from build123d import *

# Parameters (mm, degrees)
BOSS_EXTRUDE1_DEPTH      = 3
SKETCH2_W                = 13
SKETCH2_H                = 23.5
BOSS_EXTRUDE2_DEPTH      = 4
SKETCH3_W                = 6
SKETCH3_H                = 1
BOSS_EXTRUDE3_DEPTH      = 6
CHAMFER1_SIZE            = 1
SKETCH4_W                = 19
SKETCH4_H                = 29.5
BOSS_EXTRUDE4_DEPTH      = 1.5
SKETCH5_W                = 10
SKETCH5_H                = 24
CUT_EXTRUDE1_DEPTH       = 1
BOSS_EXTRUDE5_DEPTH      = 4.9
BOSS_EXTRUDE5_DEPTH_BACK = 4.9
CHAMFER2_SIZE            = 1
CHAMFER2_SIZE2           = 0.754975442


with BuildPart() as part:
    # Sketch1 → Boss-Extrude1 (new body)
    with BuildSketch(Plane(origin=(0, 0, 0), x_dir=(1, 0, 0), z_dir=(0, 1, 0))):
        Polygon((0.75, -11.75), (6.5, -11.75), (6.5, 11.75), (0.75, 11.75), (0.75, 14), (-0.75, 14), (-0.75, 11.75), (-6.5, 11.75), (-6.5, -11.75), (-0.75, -11.75), (-0.75, -14), (0.75, -14), align=None)
    extrude(amount=-BOSS_EXTRUDE1_DEPTH)

    # Sketch2 → Boss-Extrude2 (add)
    with BuildSketch(Plane.XZ.offset(3)):
        Rectangle(SKETCH2_W, SKETCH2_H)
    extrude(amount=BOSS_EXTRUDE2_DEPTH)

    # Sketch3 → Boss-Extrude3 (add)
    with BuildSketch(Plane.XZ.offset(7)):
        Rectangle(SKETCH3_W, SKETCH3_H)
        with Locations((0, 6)):
            Rectangle(SKETCH3_W, SKETCH3_H)
        with Locations((0, -6)):
            Rectangle(SKETCH3_W, SKETCH3_H)
    extrude(amount=BOSS_EXTRUDE3_DEPTH)

    # Chamfer1
    chamfer1_edges = [part.edges().sort_by_distance(p)[0] for p in [
        (-3, -13, 0),
        (3, -13, 0),
        (-3, -13, 6),
        (3, -13, 6),
        (3, -13, -6),
        (-3, -13, -6),
    ]]
    chamfer(chamfer1_edges, length=CHAMFER1_SIZE)

    # Sketch4 → Boss-Extrude4 (add)
    with BuildSketch(Plane(origin=(0, 0, 0), x_dir=(1, 0, 0), z_dir=(0, 1, 0))):
        Rectangle(SKETCH4_W, SKETCH4_H)
    extrude(amount=BOSS_EXTRUDE4_DEPTH)

    # Sketch5 → Cut-Extrude1 (cut)
    with BuildSketch(Plane(origin=(0, 1.5, 0), x_dir=(1, 0, 0), z_dir=(0, 1, 0))):
        Rectangle(SKETCH5_W, SKETCH5_H)
    extrude(amount=-CUT_EXTRUDE1_DEPTH, mode=Mode.SUBTRACT)

    # Sketch6 → Boss-Extrude5 (add, two sides: drawn at the far end of the back side and taken through both)
    with BuildSketch(Plane(origin=(0, 0, 0), x_dir=(0, 0, -1), z_dir=(1, 0, 0)).offset(-BOSS_EXTRUDE5_DEPTH_BACK)):
        Polygon((-10.977846987, 0), (10.977846987, 0), (10.977846987, 2), (0, 2), (-10.977846987, 7), align=None)
    extrude(amount=BOSS_EXTRUDE5_DEPTH + BOSS_EXTRUDE5_DEPTH_BACK)

    # Chamfer2
    chamfer2_edges = [part.edges().sort_by_distance(p)[0] for p in [
        (0, 7, 10.977846987),
    ]]
    chamfer2_side = [part.faces().sort_by_distance(p)[0] for p in [
        (0, 3.75, 10.977846987),
    ]]
    chamfer(chamfer2_edges, length=CHAMFER2_SIZE, length2=CHAMFER2_SIZE2, reference=chamfer2_side[0])


solid = part.part
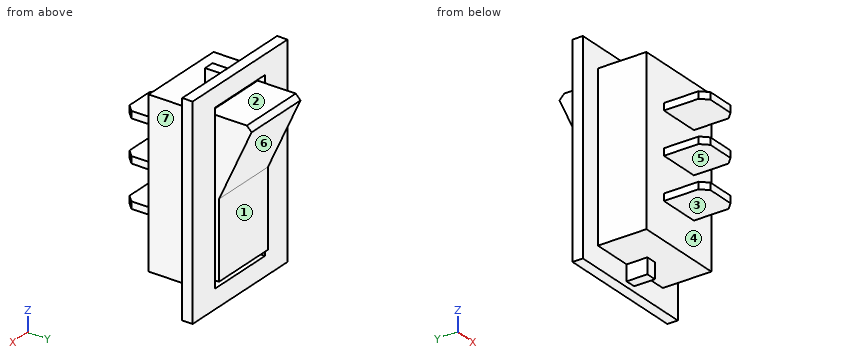
Model file for the job. Use its own axes, mm. Face numbers are marked on the shaded views. A direction names the side the tool comes from. Round coordinates to 2 decimals unless told otherwise and drop trailing zeros. Loops run counter-clockwise (first coordinate to the right, second up) from the corner with the lowest first, then second, coordinate; pieces in that order, holes last. Notation, with made-up numbers: (-20, 1.5) -> (17, 1.5) arc R20 ccw to (17, 40.5) -> close; hole circle Ø2 at (5, 79.5). An arc over 180 degrees is marked (long way). Answer as CSV lines item,"result". Start each with the question number.
1) Mould opens along Z. For the marked faces 4, 5, 6 and 7 say: +Z half, -Z half, draft (parallel to the pull), parting line (faces both ways), or undercut.
2) Slice it at D-D (y = -2.5). List the corners of the cut face in (x, z), plus the area to 3 significant figures.
3) Slice it at A-A (y = -7.75). List the corners of the cut face in (x, z), plus the area to 3 significant figures.
4) Pin check, flat tips, straight feed: P1, Ø6, axis at y = -7.5, z = -10, coming from the -X side; P2, Ø1.5, axis at y = -2.5, z = -9.5, coming from the +X side; P3, Ø5.5, axis at x = -2.5, y = -4.5, coming from the -Z side. Stop position of each tip, or through.
5) Probe line 1 along Y through (x, z) = (7.5, -2); line 2 along X through (y, z) = (-3, -6.75); line 3 along Z through (x, y) = (-0.75, -4.75). List the from-to ranges inside material, lowest first.
6) Slice it at C-C (z = -6). List the corners of the cut face in (x, y).
7) Tool access for the marked faces 1, 2 and 3: list every direction of +Z, -Z, +X, -X, +Y, -Y with a clear straight run to the whole face (end or side of a thin tool).
Filled in:
1,face 4,"undercut"
1,face 5,"undercut"
1,face 6,"-Z half"
1,face 7,"draft"
2,outline,"(-6.5, -11.75) -> (-0.75, -11.75) -> (-0.75, -14) -> (0.75, -14) -> (0.75, -11.75) -> (6.5, -11.75) -> (6.5, 11.75) -> (0.75, 11.75) -> (0.75, 14) -> (-0.75, 14) -> (-0.75, 11.75) -> (-6.5, 11.75) -> close"
2,area,"312 mm2"
3,outline,"(-3, -6.5) -> (3, -6.5) -> (3, -5.5) -> (-3, -5.5) -> close; (-3, -0.5) -> (3, -0.5) -> (3, 0.5) -> (-3, 0.5) -> close; (-3, 5.5) -> (3, 5.5) -> (3, 6.5) -> (-3, 6.5) -> close"
3,area,"18.0 mm2"
4,P1,"stops at x = -6.5"
4,P2,"stops at x = 6.5"
4,P3,"stops at z = -14"
5,line 1,"y = 0 to 1.5"
5,line 2,"x = -6.5 to 6.5"
5,line 3,"z = -11.75 to 11.75"
6,outline,"(-9.5, 0) -> (-6.5, 0) -> (-6.5, -7) -> (-3, -7) -> (-3, -12) -> (-2, -13) -> (2, -13) -> (3, -12) -> (3, -7) -> (6.5, -7) -> (6.5, 0) -> (9.5, 0) -> (9.5, 1.5) -> (5, 1.5) -> (5, 0.5) -> (4.9, 0.5) -> (4.9, 2) -> (-4.9, 2) -> (-4.9, 0.5) -> (-5, 0.5) -> (-5, 1.5) -> (-9.5, 1.5) -> close"
7,face 1,"-Z, +X, -X, +Y"
7,face 2,"+Y"
7,face 3,"-Z, +X, -X, -Y"
